Check sheet for the modelled part. Datum: model origin and axes. Units: mm. Face numbers are marked on the shaded views. A direction names the side the tool comes from. Coordinates: 2 decimals unless noted, no trailing zeros. Write each loop counter-clockwise with the first axis right and the second up, starting at its lowest first coordinate (ties: lowest second). Pieces come first, ordered by that corner, then holes. Notation, with made-up numbers: M 64.25,20 L 97.25,20 A21 cw 97.25,50 Z; hole C 65,28.5 d4. An arc over 180 degrees is marked long. Answer as CSV lines item,"result". Start each with the question number.
1) Material ranges on L1, parallel to Y at x = 0, z = 0.5; L2, parallel to Y at x = 0, z = 2.15; L3, parallel to X at y = 28.75, z = 0.4, recorded low to high. Write a range as [from, to].
2) Go/stop test with flat-tipped pins: pin 1 Ø1 at (y, z) = (26, 13) entering from +X; pin 2 Ø2 at (y, z) = (8, 24.5) entering from -X; pin 3 Ø5 at (x, z) = (19, 26.5) entering from -Y; pin 4 Ø1 at (x, y) = (-5, 24.5) entering from +Z. Record where each tip stops, or that it passes through.
3) Access from +Z, -Z, +X, -X, +Y, -Y to the whole of each face (thin tool, end or side, straight path). Record for the marked faces 1 and 2.
4) Section check A-A (z = 25.5). Record the cut outline in (x, y).
5) Section check D-D (y = 28.75). Record the cut outline in (x, z), and give its area (3 significant figures).
6) Section check B-B (y = 19). Record the cut outline in (x, z), and give its area (3 significant figures).
7) Draft check along X on the marked faces 3, 4 and 5. Enter one of: +X half, -X half, draft (parallel to the pull), parting line (faces both ways), or undercut.
8) Section check C-C (x = -4.5). Record the cut outline in (y, z), and give its area (3 significant figures).
from build123d import *

# Parameters (mm, degrees)
SKETCH1_W           = 47
SKETCH1_H           = 81.5
SKETCH1_R           = 1.75
BOSS_EXTRUDE1_DEPTH = 3.4
SKETCH2_R           = 2.8
CUT_EXTRUDE1_DEPTH  = 2.2
BOSS_EXTRUDE2_DEPTH = 2.5
BOSS_EXTRUDE3_DEPTH = 81.5
SKETCH5_R           = 2.8
CUT_EXTRUDE2_DEPTH  = 54.747674368
FILLET1_R           = 3
FILLET2_R           = 1.5


with BuildPart() as part:
    # Sketch1 → Boss-Extrude1 (new body)
    with BuildSketch(Plane.XY):
        Rectangle(SKETCH1_W, SKETCH1_H)
        with Locations((0, 28.75)):
            Circle(SKETCH1_R, mode=Mode.SUBTRACT)
        with Locations((0, -28.75)):
            Circle(SKETCH1_R, mode=Mode.SUBTRACT)
    extrude(amount=BOSS_EXTRUDE1_DEPTH)

    # Sketch2 → Cut-Extrude1 (cut)
    with BuildSketch(Plane.XY.offset(3.4)):
        with Locations((0, 28.75)):
            Circle(SKETCH2_R)
        with Locations((0, -28.75)):
            Circle(SKETCH2_R)
    extrude(amount=-CUT_EXTRUDE1_DEPTH, mode=Mode.SUBTRACT)

    # Sketch3 → Boss-Extrude2 (add)
    with BuildSketch(Plane.XY.offset(3.4)):
        Polygon((21, -38.25), (21, 38.25), (-21, 38.25), (-21, -38.25), (-21, -40.75), (-23.5, -40.75), (-23.5, 40.75), (23.5, 40.75), (23.5, -40.75), (21, -40.75), align=None)
    extrude(amount=BOSS_EXTRUDE2_DEPTH)

    # Sketch4 → Boss-Extrude3 (add)
    with BuildSketch(Plane(origin=(0, 40.75, 0), x_dir=(1, 0, 0), z_dir=(0, 1, 0))):
        with BuildLine():
            Line((23.5, -5.9), (21, -5.9))
            ThreePointArc((21, -5.9), (0, -26.9), (-21, -5.9))
            Line((-21, -5.9), (-23.5, -5.9))
            ThreePointArc((-23.5, -5.9), (0, -29.4), (23.5, -5.9))
        make_face()
    extrude(amount=-BOSS_EXTRUDE3_DEPTH)

    # Sketch5 → Cut-Extrude2 (cut, through all)
    with BuildSketch(Plane.XY.offset(3.4)):
        with Locations((0, -28.75)):
            Circle(SKETCH5_R)
        with Locations((0, 28.75)):
            Circle(SKETCH5_R)
    extrude(amount=CUT_EXTRUDE2_DEPTH, mode=Mode.SUBTRACT)

    # Fillet1
    fillet1_edges = [part.edges().sort_by_distance(p)[0] for p in [
        (-21, 39.5, 5.9),
        (21, 39.5, 5.9),
    ]]
    fillet(fillet1_edges, radius=FILLET1_R)

    # Fillet2
    fillet2_edges = [part.edges().sort_by_distance(p)[0] for p in [
        (-21, -1.25, 3.4),
        (0, 38.25, 3.4),
        (21, -1.25, 3.4),
    ]]
    fillet(fillet2_edges, radius=FILLET2_R)


solid = part.part
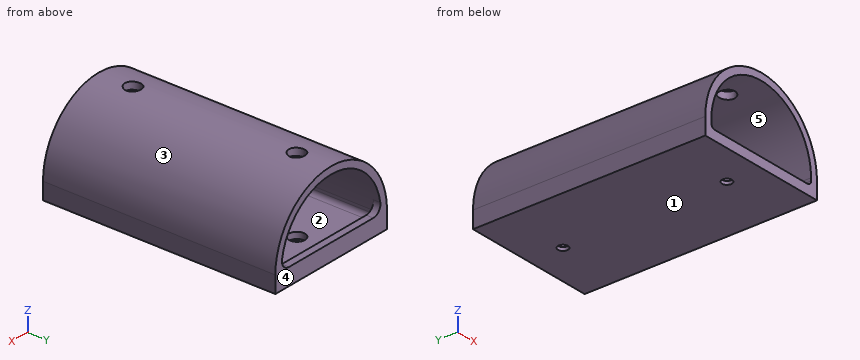
Results found:
1,L1,"y = [-40.75, -30.5], [-27, 27], [30.5, 40.75]"
1,L2,"y = [-40.75, -31.55], [-25.95, 25.95], [31.55, 40.75]"
1,L3,"x = [-23.5, -1.75], [1.75, 23.5]"
2,pin 1,"stops at x = 22.55"
2,pin 2,"stops at x = -15.57"
2,pin 3,"passes through"
2,pin 4,"stops at z = 28.97"
3,face 1,"-Z, +X, -X, +Y, -Y"
3,face 2,"-Y"
4,outline,"M -12.96,-40.75 L -7.54,-40.75 L -7.54,40.75 L -12.96,40.75 Z; M 7.54,-40.75 L 12.96,-40.75 L 12.96,40.75 L 7.54,40.75 Z"
5,outline,"M -23.5,0 L -1.75,0 L -1.75,1.2 L -2.8,1.2 L -2.8,3.4 L -19.5,3.4 A1.5 cw -21,4.9 L -21,5.9 A21 cw -2.8,26.71 L -2.8,29.23 A23.5 ccw -23.5,5.9 Z; M 1.75,0 L 23.5,0 L 23.5,5.9 A23.5 ccw 2.8,29.23 L 2.8,26.71 A21 cw 21,5.9 L 21,4.9 A1.5 cw 19.5,3.4 L 2.8,3.4 L 2.8,1.2 L 1.75,1.2 Z"
5,area,"317 mm2"
6,outline,"M -23.5,0 L 23.5,0 L 23.5,5.9 A23.5 ccw -23.5,5.9 Z; hole M -21,4.9 A1.5 ccw -19.5,3.4 L 19.5,3.4 A1.5 ccw 21,4.9 L 21,5.9 A21 ccw -21,5.9 Z"
6,area,"348 mm2"
7,face 3,"parting line"
7,face 4,"draft"
7,face 5,"undercut"
8,outline,"M -40.75,0 L 40.75,0 L 40.75,5.9 L 38.25,5.9 L 38.25,4.9 A1.5 cw 36.75,3.4 L -40.75,3.4 Z; M -40.75,26.41 L 40.75,26.41 L 40.75,28.97 L -40.75,28.97 Z"
8,area,"492 mm2"
